Can you work these out from the model? Positions are in its coordinate system, mm. Face numbers are marked on the shaded views. A direction names the side the tool comes from. Give positions to 0.01 mm unless a question says otherwise; leave off trailing zeros. Order: outer loops, then holes, each group sorted by start corner. A loop starts at its lowest first (then second) coordinate and runs counter-clockwise, first axis right, second up. Notation, with made-up numbers: (53.25, 40) -> (95.25, 40) arc R16 cw to (95.25, 50) -> close; hole circle Ø6 at (72, 21). An arc over 180 degrees is marked (long way). Answer as a JSON object with one key per item and string values.
```python
from build123d import *

# Parameters (mm, degrees)
ESBO_O1_W             = 125
ESBO_O1_H             = 124
EXTRUS_O1_DEPTH       = 3
ESBO_O2_W             = 12.7
ESBO_O2_H             = 41.5
EXTRUS_O2_DEPTH       = 9
FILETE1_R             = 4
FILETE2_R             = 2
FILETE3_R             = 4
FILETE4_R             = 2
EXTRUS_O4_START       = -3
ESBO_O3_W             = 3
ESBO_O3_H             = 10
EXTRUS_O4_DEPTH       = 38
EXTRUS_O5_DEPTH       = 150.829903557
EXTRUS_O6_DEPTH       = 150.829903557
EXTRUS_O7_DEPTH       = 3
EXTRUS_O8_DEPTH       = 3
FILETE5_R             = 4
FILETE6_R             = 4
EXTRUS_O9_DEPTH       = 3
ESBO_O10_W            = 125
ESBO_O10_H            = 4
EXTRUS_O10_DEPTH      = 13
ESBO_O11_W            = 125
ESBO_O11_H            = 3
EXTRUS_O11_DEPTH      = 40
EXTRUS_O12_DEPTH      = 40
EXTRUS_O12_DEPTH_BACK = 40
EXTRUS_O18_DEPTH      = 3
ESBO_O16_R            = 5.25
EXTRUS_O19_DEPTH      = 2


with BuildPart() as part:
    # Esboço1 → Extrusão1 (new body)
    with BuildSketch(Plane(origin=(0, 0, 0), x_dir=(1, 0, 0), z_dir=(0, 1, 0))):
        Rectangle(ESBO_O1_W, ESBO_O1_H)
    extrude(amount=EXTRUS_O1_DEPTH)

    # Esboço2 → Extrusão2 (add)
    with BuildSketch(Plane(origin=(0, 3, 0), x_dir=(1, 0, 0), z_dir=(0, 1, 0))):
        Polygon((-62.5, -26), (-62.5, -14.5), (-43.8, -14.5), (-43.8, -62), (-62.5, -62), (-62.5, -36), align=None)
        with Locations((-53.15, -38.25)):
            Rectangle(ESBO_O2_W, ESBO_O2_H, mode=Mode.SUBTRACT)
    extrus_o2 = extrude(amount=EXTRUS_O2_DEPTH)

    # Filete1
    filete1_edges = [part.edges().sort_by_distance(p)[0] for p in [
        (-62.5, 7.5, 14.5),
        (-43.8, 7.5, 14.5),
    ]]
    fillet(filete1_edges, radius=FILETE1_R)

    # Filete2
    filete2_edges = [part.edges().sort_by_distance(p)[0] for p in [
        (-46.8, 7.5, 17.5),
        (-59.5, 7.5, 17.5),
    ]]
    fillet(filete2_edges, radius=FILETE2_R)

    # Espelhar3: Extrusão2 across plane
    add(extrus_o2.mirror(Plane(origin=(0, 0, 0), x_dir=(0, 0, 1), z_dir=(1, 0, 0))))

    # Filete3
    filete3_edges = [part.edges().sort_by_distance(p)[0] for p in [
        (62.5, 7.5, 14.5),
        (43.8, 7.5, 14.5),
    ]]
    fillet(filete3_edges, radius=FILETE3_R)

    # Filete4
    filete4_edges = [part.edges().sort_by_distance(p)[0] for p in [
        (59.5, 7.5, 17.5),
        (46.8, 7.5, 17.5),
    ]]
    fillet(filete4_edges, radius=FILETE4_R)

    # Esboço3 → Extrusão4 (add)
    with BuildSketch(Plane(origin=(0, 3, 0), x_dir=(1, 0, 0), z_dir=(0, 1, 0)).offset(EXTRUS_O4_START)):
        with Locations((-64, -31)):
            Rectangle(ESBO_O3_W, ESBO_O3_H)
        with Locations((-42.3, -31)):
            Rectangle(ESBO_O3_W, ESBO_O3_H)
    extrus_o4 = extrude(amount=EXTRUS_O4_DEPTH)

    # Espelhar6: Extrusão4 across plane
    add(extrus_o4.mirror(Plane(origin=(0, 0, 0), x_dir=(0, 0, 1), z_dir=(1, 0, 0))))

    # Esboço5 → Extrusão5 (cut, through all)
    with BuildSketch(Plane.ZY.offset(65.5)):
        with BuildLine():
            Line((30.5, 12), (31.5, 12))
            ThreePointArc((31.5, 12), (32.560660172, 12.439339828), (33, 13.5))
            Line((33, 13.5), (33, 15.5))
            ThreePointArc((33, 15.5), (32.560660172, 16.560660172), (31.5, 17))
            Line((31.5, 17), (30.5, 17))
            ThreePointArc((30.5, 17), (29.439339828, 16.560660172), (29, 15.5))
            Line((29, 15.5), (29, 13.5))
            ThreePointArc((29, 13.5), (29.439339828, 12.439339828), (30.5, 12))
        make_face()
    extrude(amount=-EXTRUS_O5_DEPTH, mode=Mode.SUBTRACT)

    # Esboço6 → Extrusão6 (cut, through all)
    with BuildSketch(Plane.ZY.offset(65.5)):
        with BuildLine():
            Line((30.5, 30), (31.5, 30))
            ThreePointArc((31.5, 30), (32.560660172, 30.439339828), (33, 31.5))
            Line((33, 31.5), (33, 33.5))
            ThreePointArc((33, 33.5), (32.560660172, 34.560660172), (31.5, 35))
            Line((31.5, 35), (30.5, 35))
            ThreePointArc((30.5, 35), (29.439339828, 34.560660172), (29, 33.5))
            Line((29, 33.5), (29, 31.5))
            ThreePointArc((29, 31.5), (29.439339828, 30.439339828), (30.5, 30))
        make_face()
    extrude(amount=-EXTRUS_O6_DEPTH, mode=Mode.SUBTRACT)

    # Esboço7 → Extrusão7 (add)
    with BuildSketch(Plane.ZY.offset(65.5)):
        Polygon((26, 0), (22, 0), (26, 38), align=None)
        Polygon((36, 38), (36, 0), (40, 0), align=None)
    extrus_o7 = extrude(amount=-EXTRUS_O7_DEPTH)

    # Esboço8 → Extrusão8 (add)
    with BuildSketch(Plane.ZY.offset(43.8)):
        Polygon((26, 38), (22, 0), (26, 0), align=None)
        Polygon((36, 38), (36, 0), (40, 0), align=None)
    extrus_o8 = extrude(amount=-EXTRUS_O8_DEPTH)

    # Filete5
    filete5_edges = [part.edges().sort_by_distance(p)[0] for p in [
        (-64, 38, 26),
        (-64, 38, 36),
        (-42.3, 38, 36),
        (-42.3, 38, 26),
    ]]
    fillet(filete5_edges, radius=FILETE5_R)

    # Espelhar9: Extrusão7, Extrusão8 across plane
    add(extrus_o7.mirror(Plane(origin=(0, 0, 0), x_dir=(0, 0, 1), z_dir=(1, 0, 0))))
    add(extrus_o8.mirror(Plane(origin=(0, 0, 0), x_dir=(0, 0, 1), z_dir=(1, 0, 0))))

    # Filete6
    filete6_edges = [part.edges().sort_by_distance(p)[0] for p in [
        (64, 38, 26),
        (64, 38, 36),
        (42.3, 38, 36),
        (42.3, 38, 26),
    ]]
    fillet(filete6_edges, radius=FILETE6_R)

    # Esboço9 → Extrusão9 (cut)
    with BuildSketch(Plane(origin=(0, 3, 0), x_dir=(1, 0, 0), z_dir=(0, 1, 0))):
        with BuildLine():
            Line((-12.5, -17.5), (12.5, -17.5))
            ThreePointArc((12.5, -17.5), (14.267766953, -16.767766953), (15, -15))
            Line((15, -15), (15, 10))
            ThreePointArc((15, 10), (14.267766953, 11.767766953), (12.5, 12.5))
            Line((12.5, 12.5), (-12.5, 12.5))
            ThreePointArc((-12.5, 12.5), (-14.267766953, 11.767766953), (-15, 10))
            Line((-15, 10), (-15, -15))
            ThreePointArc((-15, -15), (-14.267766953, -16.767766953), (-12.5, -17.5))
        make_face()
    extrude(amount=-EXTRUS_O9_DEPTH, mode=Mode.SUBTRACT)

    # Esboço10 → Extrusão10 (add)
    with BuildSketch(Plane(origin=(0, 3, 0), x_dir=(1, 0, 0), z_dir=(0, 1, 0))):
        with Locations((0, 60)):
            Rectangle(ESBO_O10_W, ESBO_O10_H)
    extrude(amount=EXTRUS_O10_DEPTH)

    # Esboço11 → Extrusão11 (add)
    with BuildSketch(Plane(origin=(0, 0, -62), x_dir=(-1, 0, 0), z_dir=(0, 0, -1))):
        with Locations((0, 14.5)):
            Rectangle(ESBO_O11_W, ESBO_O11_H)
    extrude(amount=EXTRUS_O11_DEPTH)

    # Esboço13 → Extrusão12 (cut, two sides: drawn at the far end of the back side and taken through both)
    with BuildSketch(Plane(origin=(0, 3, 0), x_dir=(1, 0, 0), z_dir=(0, 1, 0)).offset(-EXTRUS_O12_DEPTH_BACK)):
        Polygon((-62.5, 3), (-27.5, 102), (-62.5, 102), align=None)
        Polygon((27.5, 102), (62.5, 102), (62.5, 3), align=None)
    extrude(amount=EXTRUS_O12_DEPTH + EXTRUS_O12_DEPTH_BACK, mode=Mode.SUBTRACT)

    # Esboço15 → Extrusão18 (add)
    with BuildSketch(Plane(origin=(56.498957011, 0, -19.974378741), x_dir=(-0.3333182172036595, 0, -0.9428143858046366), z_dir=(0.9428143858046366, 0, -0.3333182172036595))):
        Polygon((44.72381831, 16), (40.332033358, 16), (-18.003945418, 3), (-18.003945418, 0), (44.574649996, 0), align=None)
    extrus_o18 = extrude(amount=-EXTRUS_O18_DEPTH)

    # Espelhar10: Extrusão18 across plane
    add(extrus_o18.mirror(Plane(origin=(0, 0, 0), x_dir=(0, 0, 1), z_dir=(1, 0, 0))))

    # Esboço16 → Extrusão19 (cut)
    with BuildSketch(Plane.XZ):
        with Locations(Location((-12, 52, 0), (0, 0, 270))):
            Circle(ESBO_O16_R)
        with Locations(Location((12, 52, 0), (0, 0, 270))):
            Circle(ESBO_O16_R)
        with Locations(Location((-12, -47, 0), (0, 0, 270))):
            Circle(ESBO_O16_R)
        with Locations(Location((12, -47, 0), (0, 0, 270))):
            Circle(ESBO_O16_R)
    extrude(amount=-EXTRUS_O19_DEPTH, mode=Mode.SUBTRACT)


solid = part.part
```
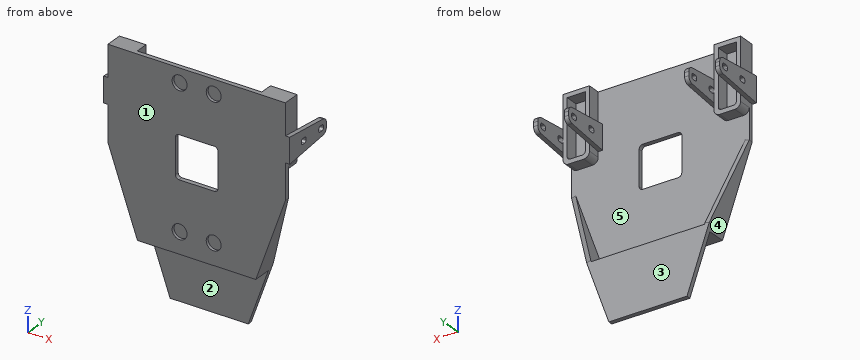
1. If we section it at B-B on y = 27: Please give me the cut outline in (x, z), then the cut area to 3 significant figures.
Worked answers:
{"outline": "(-65.5, 24.84) -> (-62.5, 24.84) -> (-62.5, 37.16) -> (-65.5, 37.16) -> close; (-43.8, 24.84) -> (-40.8, 24.84) -> (-40.8, 37.16) -> (-43.8, 37.16) -> close; (40.8, 24.84) -> (43.8, 24.84) -> (43.8, 37.16) -> (40.8, 37.16) -> close; (62.5, 24.84) -> (65.5, 24.84) -> (65.5, 37.16) -> (62.5, 37.16) -> close", "area": "148 mm²"}
2. If we section it at A-A on z = 10: Please give me the cut outline in (x, y), then the cut area to 3 significant figures.
Worked answers:
{"outline": "(-62.5, 0) -> (-15, 0) -> (-15, 3) -> (-62.5, 3) -> close; (15, 0) -> (62.5, 0) -> (62.5, 3) -> (15, 3) -> close", "area": "285 mm²"}
3. Please list where these lines run through material, in increasing order: L1, parallel to X at y = 0.8, z = 52; L2, parallel to X at y = 29, z = 32.5; L3, parallel to Y at x = -16.5, z = 34.5.
Worked answers:
{"L1": "-62.5 to -17.25, -6.75 to 6.75, 17.25 to 62.5", "L2": "-65.5 to -62.5, -43.8 to -40.8, 40.8 to 43.8, 62.5 to 65.5", "L3": "0 to 3"}
4. If we section it at C-C on x = -35: Please give me the cut outline in (y, z).
Worked answers:
{"outline": "(0, -62) -> (13, -62) -> (13, -80.79) -> (16, -80.79) -> (16, -58) -> (3, -58) -> (3, 62) -> (0, 62) -> close"}
5. If we section it at D-D on z = -47: Please give me the cut outline in (x, y).
Worked answers:
{"outline": "(-46.94, 0) -> (-17.25, 0) -> (-17.25, 2) -> (-6.75, 2) -> (-6.75, 0) -> (6.75, 0) -> (6.75, 2) -> (17.25, 2) -> (17.25, 0) -> (46.94, 0) -> (46.94, 13.4) -> (43.76, 13.64) -> (43.76, 3) -> (-43.76, 3) -> (-43.76, 13.64) -> (-46.94, 13.4) -> close"}
6. For the marked faces 1 and 2, which set-ups out of +Z, -Z, +X, -X, +Y, -Y let a thin tool reach every point of the face, with its end or its side?
Worked answers:
{"face 1": "+Z, -Z, +X, -X, -Y", "face 2": "-Z, +X, -X, -Y"}
7. Will these pins go through, and if not, where does the flat tip stop? pin 1 Ø6.5 at (x, z) = (-54.5, 48) entering from +Y; pin 2 Ø20 at (x, z) = (-53, 29) entering from +Y; pin 3 Ø8 at (x, y) = (-13, 19.5) entering from +Z; pin 4 Ø5 at (x, y) = (-40.5, 24.5) entering from +Z.
Worked answers:
{"pin 1": "y = 3", "pin 2": "y = 38", "pin 3": "z = -58", "pin 4": "z = 37.68"}
8. If we mould it in two halves opening along X, with no side actions, what happens to the marked faces 3, 4 and 5? For each: +X half, -X half, draft (parallel to the pull), parting line (faces both ways), or undercut.
Worked answers:
{"face 3": "draft", "face 4": "-X half", "face 5": "undercut"}
